Verification items for the finished model (mm, model axes). Round coordinates to 2 decimals unless told otherwise and drop trailing zeros. Order: outer loops, then holes, each group sorted by start corner. A loop starts at its lowest first (then second) coordinate and runs counter-clockwise, first axis right, second up. Notation, with made-up numbers: (47, 41) -> (69, 41) arc R30 cw to (69, 76) -> close; hole circle Ø10 at (36.25, -7.5). An arc over 180 degrees is marked (long way). Put each result on its own line as item: value.
Autodesk Inventor part; units mm, degrees
ref_plane "YZ Plane" through (0, 0, 0) normal (1, 0, 0) x (0, 1, 0)
ref_plane "XZ Plane" through (0, 0, 0) normal (0, 1, 0) x (-1, 0, 0)
ref_plane "XY Plane" through (0, 0, 0) normal (0, 0, 1) x (1, 0, 0)
sketch "Эскиз2" plane through (0, 0, 0) normal (0, 1, 0) x (-1, 0, 0)
  line L0 (0, 26) -> (0, -26) construction
  arc A0 (-12.5, 26) -> (-12.1796, 28.8119) centre (0, 26) ccw construction
  line L1 (0, 26) -> (5.8487, 51.3336) construction
  arc A1 (18.0284, 48.5217) -> (-6.3309, 54.1455) centre (5.8487, 51.3336) ccw
  line L2 (0, 0) -> (59.5469, 0) construction
  line L3 (18.0284, 48.5217) -> (12.1796, 23.1881)
  line L4 (-6.3309, 54.1455) -> (-11.682, 30.9675)
  arc A2 (3.0368, 39.154) -> (18.0284, 48.5217) centre (5.8487, 51.3336) ccw construction
  arc A3 (-6.3309, 54.1455) -> (3.0368, 39.154) centre (5.8487, 51.3336) ccw construction
  arc A4 (-12.1796, -28.8119) -> (-12.5, -26) centre (0, -26) ccw construction
  arc A5 (-6.3309, -54.1455) -> (18.0284, -48.5217) centre (5.8487, -51.3336) ccw
  line L5 (18.0284, -48.5217) -> (12.1796, -23.1881)
  line L6 (-6.3309, -54.1455) -> (-11.682, -30.9675)
  arc A6 (18.0284, -48.5217) -> (3.0368, -39.154) centre (5.8487, -51.3336) ccw construction
  arc A7 (3.0368, -39.154) -> (-6.3309, -54.1455) centre (5.8487, -51.3336) ccw construction
  line L7 (12.1796, 23.1881) -> (12.1796, -23.1881)
  arc A8 (-12.1796, 28.8119) -> (-12.5, 26) centre (0, 26) ccw construction
  arc A9 (-12.5, -26) -> (-12.1796, -28.8119) centre (0, -26) ccw construction
  line L8 (-18, 17) -> (-18, -17) construction
  circle A10 centre (-18, 17) radius 1.5
  circle A11 centre (-18, -17) radius 1.5
  arc A12 (-20.8814, 19.7744) -> (-22, 17) centre (-18, 17) ccw
  arc A13 (-18, -13) -> (-22, -17) centre (-18, -17) ccw construction
  line L9 (-22, 17) -> (-22, -17)
  line L10 (-20.8814, 19.7744) -> (-13.7141, 27.2183)
  arc A14 (-13.7141, 27.2183) -> (-11.682, 30.9675) centre (-19.4769, 32.7671) ccw
  arc A15 (-18, 13) -> (-20.8814, 19.7744) centre (-18, 17) ccw construction
  arc A16 (-22, 17) -> (-18, 13) centre (-18, 17) ccw construction
  arc A17 (-22, -17) -> (-20.8814, -19.7744) centre (-18, -17) ccw
  line L11 (-13.7141, -27.2183) -> (-20.8814, -19.7744)
  arc A18 (-11.682, -30.9675) -> (-13.7141, -27.2183) centre (-19.4769, -32.7671) ccw
  arc A19 (-20.8814, -19.7744) -> (-18, -13) centre (-18, -17) ccw construction
  circle A20 centre (-4.794, 0) radius 5
  point P0 (-18, 0)
  point P1 (0, 0)
  dimension "d14" = 52
  dimension "d15" = 26
  dimension "d16" = 25
  dimension "d17" = 26
  dimension "d18" = 167
  dimension "d19" = 25
  dimension "d20" = 34
  dimension "d21" = 18
  dimension "d22" = 3
  dimension "d23" = 3
  dimension "d24" = 8
  dimension "d25" = 8
  dimension "d26" = 8
  dimension "d27" = 8
  dimension "d28" = 10
  dimension "d29" = 4.794
  dimension "d32" = 26
  dimension "d33" = 51.3336
  dimension "d34" = 4.794
  dimension "d35" = 10.6427
extrude "Выдавливание2" add sketch "Эскиз2" along normal blind 1.5
properties part number "Capasitor_board"
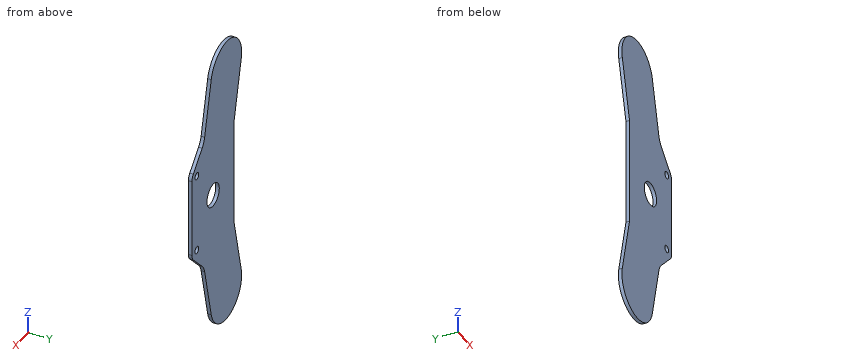
Item 1: Sectioned sample at A-A, the plane z = 0. Record the boundary of the cut face in (x, y), then the cut area to 3 significant figures.
Geometry check:
outline: (-12.18, 0) -> (-0.21, 0) -> (-0.21, 1.5) -> (-12.18, 1.5) -> close; (9.79, 0) -> (22, 0) -> (22, 1.5) -> (9.79, 1.5) -> close
area: 36.3 mm2
Item 2: Sectioned sample at C-C, the plane y = 0.25. Record the boundary of the cut face in (x, z).
Geometry check:
outline: (-18.03, -48.52) arc R12.5 ccw to (6.33, -54.15) -> (11.68, -30.97) arc R8 cw to (13.71, -27.22) -> (20.88, -19.77) arc R4 ccw to (22, -17) -> (22, 17) arc R4 ccw to (20.88, 19.77) -> (13.71, 27.22) arc R8 cw to (11.68, 30.97) -> (6.33, 54.15) arc R12.5 ccw to (-18.03, 48.52) -> (-12.18, 23.19) -> (-12.18, -23.19) -> close; hole circle Ø10 at (4.79, 0); hole circle Ø3 at (18, -17); hole circle Ø3 at (18, 17)
Item 3: Material ranges on line 1 along Z through (x, y) = (18, 0.55); line 2 along X through (y, z) = (1.05, 3.5); line 3 along X through (y, z) = (1.1, -11.5), recorded low to high.
Geometry check:
line 1: -22.77 to -18.5, -15.5 to 15.5, 18.5 to 22.77
line 2: -12.18 to 1.22, 8.36 to 22
line 3: -12.18 to 22
Item 4: Sectioned sample at B-B, the plane x = 18. Record the boundary of the cut face in (y, z).
Geometry check:
outline: (0, -22.77) -> (1.5, -22.77) -> (1.5, -18.5) -> (0, -18.5) -> close; (0, -15.5) -> (1.5, -15.5) -> (1.5, 15.5) -> (0, 15.5) -> close; (0, 18.5) -> (1.5, 18.5) -> (1.5, 22.77) -> (0, 22.77) -> close
Item 5: Sectioned sample at D-D, the plane x = 2.5. Record the boundary of the cut face in (y, z).
Geometry check:
outline: (0, -60.64) -> (1.5, -60.64) -> (1.5, -4.44) -> (0, -4.44) -> close; (0, 4.44) -> (1.5, 4.44) -> (1.5, 60.64) -> (0, 60.64) -> close
